Check sheet for the modelled part. Datum: model origin and axes. Units: mm. A direction names the side the tool comes from. Coordinates: 2 decimals unless noted, no trailing zeros. Loops run counter-clockwise (first coordinate to the right, second up) from the corner with the lowest first, then second, coordinate; pieces in that order, holes last.
```python
from build123d import *

# Parameters (mm, degrees)
F1_DEPTH  = 16
F2_W      = 70
F2_H      = 3
F3_DEPTH  = 2
F4_W      = 52.4458656609
F4_H      = 13.8459985778
F5_DEPTH  = 2
F8_DEPTH  = 2
F9_R      = 2
F11_DEPTH = 38.001
F13_D     = 4
F14_R     = 3
F14_R_2   = 2
F15_DEPTH = 34.5


with BuildPart() as f1:
    # F0 (on Front) → F1 (new body)
    with BuildSketch(Plane.XZ):
        with BuildLine():
            Line((94, 9), (0, 9))
            ThreePointArc((0, 9), (-9, 0), (0, -9))
            Line((0, -9), (10, -9))
            ThreePointArc((10, -9), (12.1096761181, -9.4668701015), (13.8253743549, -10.7802933293))
            ThreePointArc((13.8253743549, -10.7802933293), (34.9359413113, -40.7908803671), (68.327168476, -56))
            ThreePointArc((68.327168476, -56), (81.3946239912, -51.9695299334), (91.6636888451, -61))
            Line((91.6636888451, -61), (93.1092569516, -59.2209782))
            ThreePointArc((93.1092569516, -59.2209782), (81.7616044026, -50.0028575081), (67.6586675506, -53.8564453964))
            ThreePointArc((67.6586675506, -53.8564453964), (35.7039452814, -38.8251123565), (15.5964314226, -9.7952461033))
            ThreePointArc((15.5964314226, -9.7952461033), (13.1278365305, -7.7376810494), (10, -7))
            Line((10, -7), (0, -7))
            ThreePointArc((0, -7), (-7, 0), (0, 7))
            Line((0, 7), (94, 7))
            Line((94, 7), (94, 9))
        make_face()
    extrude(amount=F1_DEPTH)

    # F2 (on face) → F3 (join)
    with BuildSketch(Plane.XY.offset(9)):
        with Locations((59, -17.5)):
            Rectangle(F2_W, F2_H)
    extrude(amount=-F3_DEPTH)

    # F4 (on face) → F5 (join)
    with BuildSketch(Plane.XZ.offset(19)):
        with Locations((67.7770671695, 0.0770007111)):
            Rectangle(F4_W, F4_H)
    extrude(amount=-F5_DEPTH)

    # F6: F1 across face


with BuildPart() as f1_1:
    add(f1.part)
    add(f1.part.mirror(Plane(origin=(40.1817011291, 0, -15.4832521129), x_dir=(1, 0, 0), z_dir=(0, 1, 0))))

    # F7 (on face) → F8 (cut)
    with BuildSketch(Plane.XY.offset(9)):
        with BuildLine():
            Line((34, -10.5), (94, -10.5))
            Line((94, -10.5), (94, 10.5))
            Line((94, 10.5), (34, 10.5))
            ThreePointArc((34, 10.5), (27.8094750193, 0), (34, -10.5))
        make_face()
    extrude(amount=-F8_DEPTH, mode=Mode.SUBTRACT)

    # F9
    f9_edges = [f1_1.edges().sort_by_distance(p)[0] for p in [
        (59, -19, 9),
        (59, 19, 9),
    ]]
    fillet(f9_edges, radius=F9_R)

    # F10 (on face) → F11 (cut, through all)
    with BuildSketch(Plane.XZ.offset(19)):
        with BuildLine():
            ThreePointArc((70.0115500211, -2.922977055), (72.9999777661, 0.0885507322), (69.9884499789, 3.0769784772))
            Line((69.9884499789, 3.0769784772), (49.9884499789, 2.9999777661))
            ThreePointArc((49.9884499789, 2.9999777661), (47.0000222339, -0.0115500211), (50.0115500211, -2.9999777661))
            Line((50.0115500211, -2.9999777661), (70.0115500211, -2.922977055))
        make_face()
    extrude(amount=-F11_DEPTH, mode=Mode.SUBTRACT)

    # F13 (through all)
    with Locations(Plane(origin=(0, 19, 0), x_dir=(-1, 0, 0), z_dir=(0, 1, 0))):
        with Locations((-80, -0.8459985778)):
            Hole(F13_D / 2)

    # F14 (on face) → F15 (join)
    with BuildSketch(Plane(origin=(0, -17, 0), x_dir=(-1, 0, 0), z_dir=(0, 1, 0))):
        with Locations((-80, -0.8459985778)):
            Circle(F14_R)
        with Locations((-80, -0.8459985778)):
            Circle(F14_R_2, mode=Mode.SUBTRACT)
    extrude(amount=F15_DEPTH)


solid = f1_1.part
```
1) Mould release check, pull along Z, two halves, no side actions. Record for faces 6 (the cylindrical face through (59.49, 18.43, 8.4)), 7 (the flat face through (67, 18, -6.846)), 8 (the cylindrical face through (73, -18, 0)): +Z half, -Z half, draft (parallel to the pull), parting line (faces both ways), or undercut.
Answer sheet:
face 6: +Z half
face 7: -Z half
face 8: undercut
2) Section check B-B on z = 5.5. Enter the section's corners in (x, y).
Answer sheet:
outline: (-7.12, -16) - (-4.33, -16) - (-4.33, 16) - (-7.12, 16) - close; (41.55, -19) - (94, -19) - (94, -17) - (41.55, -17) - close; (41.55, 17) - (94, 17) - (94, 19) - (41.55, 19) - close
3) Set-up check for faces 1 (the flat face through (5, 0, -7)), 2 (the cylindrical face through (82.997, -0.238, -0.714)), 3 (the flat face through (24, 17, 8)), 4 (the flat face through (41.554, 18, 0)), 5 (the flat face through (23, 16, -26)): record each of +Z, -Z, +X, -X, +Y, -Y from which the full face is reachable in a straight line by a thin tool's end or side.
Answer sheet:
face 1: +X, +Y, -Y
face 2: none
face 3: +Z, -Z, -X, +Y
face 4: -Z, -X, +Y, -Y
face 5: -Z, -X, +Y
4) Depth check by flat-ended pin: pin 1 (1.6 mm diameter, centred on x = 51, z = 8.5, fed in from +Y); pin 2 (6.5 mm diameter, centred on x = 80, z = -0.85, fed in from -Y); pin 3 (4 mm diameter, centred on y = 4, z = -15.5, fed in from -X); pin 4 (12 mm diameter, centred on y = -12, z = -19.5, fed in from +X). Enter the tip coordinate at first touch or a pass-through.
Answer sheet:
pin 1: stops at y = 18.87
pin 2: stops at y = -19
pin 3: stops at x = 14.88
pin 4: stops at x = 23.64
5) Section check A-A on x = 80. Enter the section's corners in (y, z), plus the area to 3 significant figures.
Answer sheet:
outline: (-19, -6.85) - (-17, -6.85) - (-17, -3.85) - (17, -3.85) - (17, -6.85) - (19, -6.85) - (19, -2.85) - (-19, -2.85) - close; (-19, 1.15) - (19, 1.15) - (19, 7) arc R2 ccw to (17, 9) - (10.5, 9) - (10.5, 7) - (17, 7) - (17, 2.15) - (-17, 2.15) - (-17, 7) - (-10.5, 7) - (-10.5, 9) - (-17, 9) arc R2 ccw to (-19, 7) - close; (-16, -51.74) - (16, -51.74) - (16, -49.73) - (-16, -49.73) - close
area: 204 mm2
6) Section check D-D on z = -35. Enter the section's corners in (x, y).
Answer sheet:
outline: (28.76, -16) - (31.55, -16) - (31.55, 16) - (28.76, 16) - close
7) Section check C-C on x = 54. Enter the section's corners in (y, z), plus the area to 3 significant figures.
Answer sheet:
outline: (-19, -6.85) - (-17, -6.85) - (-17, -2.98) - (-19, -2.98) - close; (-19, 3.02) - (-17, 3.02) - (-17, 7) - (-10.5, 7) - (-10.5, 9) - (-17, 9) arc R2 ccw to (-19, 7) - close; (-16, -52.06) - (16, -52.06) - (16, -49.9) - (-16, -49.9) - close; (10.5, 7) - (17, 7) - (17, 3.02) - (19, 3.02) - (19, 7) arc R2 ccw to (17, 9) - (10.5, 9) - close; (17, -6.85) - (19, -6.85) - (19, -2.98) - (17, -2.98) - close
area: 133 mm2
8) Scan lines: line 1 (Z direction, x = 4.5, y = 5.5); line 2 (X direction, y = 10, z = 0.5); line 3 (Y direction, x = 76, z = 0). Record each from-to range of solid material in increasing order.
Answer sheet:
line 1: z = -9 to -7, 7 to 9
line 2: x = -8.99 to -6.98, 77.32 to 78.52, 81.48 to 82.68
line 3: y = -19 to -17, 17 to 19
